Could you check a few things on this drawing? It's one solid part, dimensions in mm from its lowest x, y, z. A direction names the side the tool comes from. Round coordinates to 2 decimals unless told otherwise and drop trailing zeros. Write each loop counter-clockwise with the first axis right and the second up, starting at its lowest first coordinate (ties: lowest second). Pieces come first, ordered by that corner, then holes. Notation, with made-up numbers: (38.5, 40.25) -> (75.5, 40.25) arc R14 cw to (75.5, 63.25) -> close; hole circle Ø9 at (3, 5.5). An arc over 180 degrees is marked (long way). Answer in a Markdown table with one row per item. Add a question column.
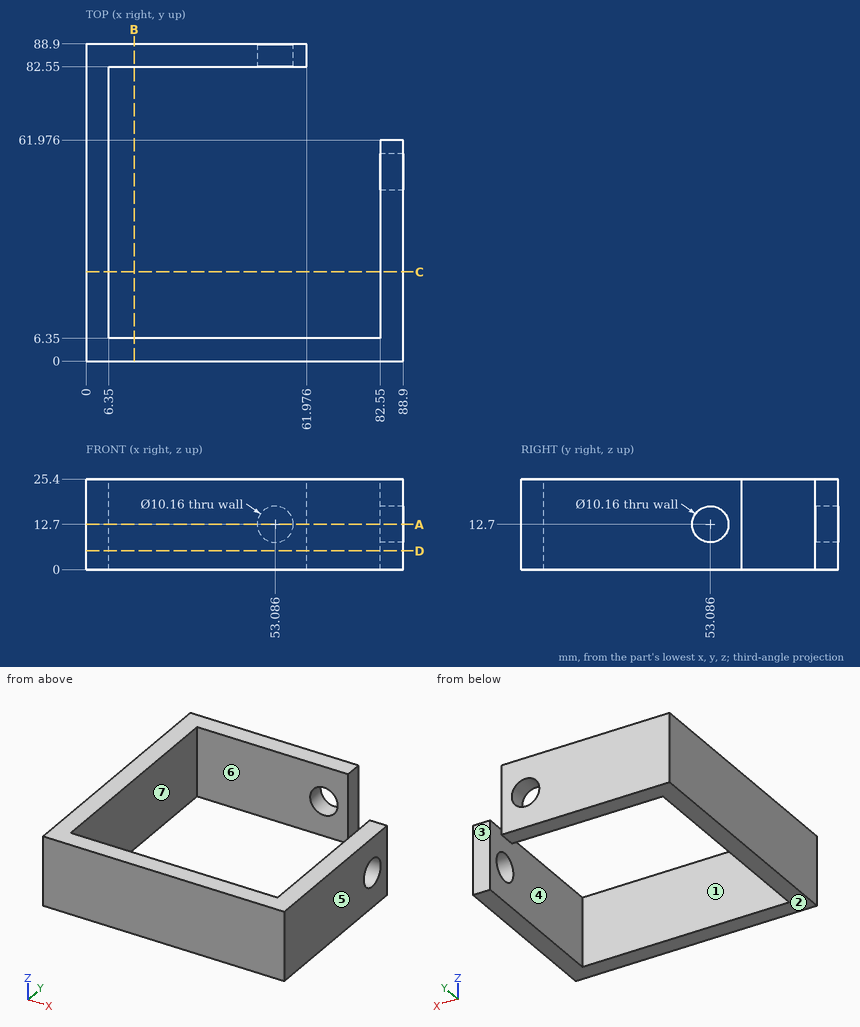
Item 1: If we section it at A-A on z = 12.7: Please give me the cut outline in (x, y), then the cut area to 3 significant figures.
Item 2: I need wall thicknesses on line 1 along X through (y, z) = (32.5, 7.5); line 2 along Y through (x, z) = (80, 9.5). Which ranges of each line are inside material? Lowest first, please. Write a range as from..to.
Item 3: On a 3-axis mill with a long thin cutter (end or side, diameter ignored), from which of +Z, -Z, +X, -X, +Y, -Y can I reach the whole of each face in a straight line? I mean the marked faces 1, 2 and 3. Say none if no direction works.
Item 4: If we section it at B-B on x = 13.5: Please give me the cut outline in (y, z), then the cut area to 3 significant figures.
Item 5: If we section it at D-D on z = 5.25: Please give me the cut outline in (x, y), then the cut area to 3 significant figures.
Item 6: For P1, Ø9, axis at x = 53.086, z = 12.7, coming from the +Y side; P2, Ø3, axis at x = 85, z = 9, coming from the +Y side; P3, Ø5, axis at y = 86, z = 14, coming from the +X side, each with a flat end and sliding along its axis, tell me the tip position at first contact or that it passes through.
Item 7: If we mould it in two halves opening along X, with no side actions, what happens to the marked faces 4, 5, 6 and 7? For each: pulls with the +X half, pulls with the -X half, needs draft (parallel to the pull), parting line crosses it, or undercut.
Results list:
| question | item | result |
|---|---|---|
| 1 | outline | (0, 0) -> (88.9, 0) -> (88.9, 48.01) -> (82.55, 48.01) -> (82.55, 6.35) -> (6.35, 6.35) -> (6.35, 82.55) -> (48.01, 82.55) -> (48.01, 88.9) -> (0, 88.9) -> close; (58.17, 82.55) -> (61.98, 82.55) -> (61.98, 88.9) -> (58.17, 88.9) -> close; (82.55, 58.17) -> (88.9, 58.17) -> (88.9, 61.98) -> (82.55, 61.98) -> close |
| 1 | area | 1,670 mm² |
| 2 | line 1 | 0..6.35, 82.55..88.9 |
| 2 | line 2 | 0..6.35 |
| 3 | face 1 | +Z, -Z |
| 3 | face 2 | -Z, +X, -X, +Y, -Y |
| 3 | face 3 | +Z, -Z, +X, +Y |
| 4 | outline | (0, 0) -> (6.35, 0) -> (6.35, 25.4) -> (0, 25.4) -> close; (82.55, 0) -> (88.9, 0) -> (88.9, 25.4) -> (82.55, 25.4) -> close |
| 4 | area | 323 mm² |
| 5 | outline | (0, 0) -> (88.9, 0) -> (88.9, 61.98) -> (82.55, 61.98) -> (82.55, 6.35) -> (6.35, 6.35) -> (6.35, 82.55) -> (61.98, 82.55) -> (61.98, 88.9) -> (0, 88.9) -> close |
| 5 | area | 1,800 mm² |
| 6 | P1 | y = 6.35 |
| 6 | P2 | y = 61.98 |
| 6 | P3 | x = 61.98 |
| 7 | face 4 | undercut |
| 7 | face 5 | pulls with the +X half |
| 7 | face 6 | needs draft |
| 7 | face 7 | undercut |
